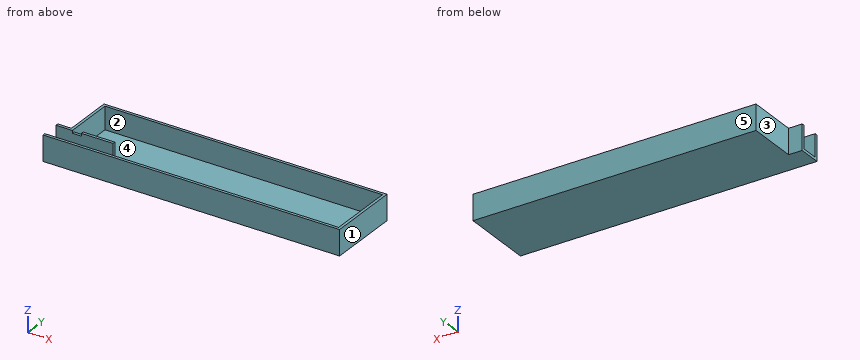
from build123d import *

# Parameters (mm, degrees)
F1_DEPTH = 1.2
F2_W     = 18
F2_H     = 1.2
F3_DEPTH = 10
F4_W     = 4
F4_H     = 1.2
F5_DEPTH = 1.2


with BuildPart() as f1:
    # F0 (on Top) → F1 (new body)
    with BuildSketch(Plane.XY):
        Polygon((-125, 0), (0, 0), (0, 32), (-125, 32), (-125, 10), (-131, 10), (-131, 0), align=None)
    extrude(amount=F1_DEPTH)

    # F2 (on face) → F3 (join)
    with BuildSketch(Plane.XY.offset(1.2)):
        Polygon((-131, 0), (0, 0), (0, 32), (-125, 32), (-125, 10), (-131, 10), (-131, 8.8), (-123.8, 8.8), (-123.8, 10), (-123.8, 30.8), (-1.2, 30.8), (-1.2, 1.2), (-131, 1.2), align=None)
        with Locations((-114.8, 9.4)):
            Rectangle(F2_W, F2_H)
    extrude(amount=F3_DEPTH)

    # F4 (on face) → F5 (cut, through all)
    with BuildSketch(Plane(origin=(0, 10, 0), x_dir=(-1, 0, 0), z_dir=(0, 1, 0))):
        with Locations((121.8, 10.6)):
            Rectangle(F4_W, F4_H)
    extrude(amount=-F5_DEPTH, mode=Mode.SUBTRACT)


solid = f1.part
For this review, take the finished solid that the model builds, in its own axes (mm). Face numbers are marked on the shaded views. A direction names the side the tool comes from. Give positions to 0.01 mm unless a question says otherwise; leave off trailing zeros. Loops run counter-clockwise (first coordinate to the right, second up) from the corner with the lowest first, then second, coordinate; pieces in that order, holes last.
Item 1: Take a section at B-B, the plane y = 15.5. State the section outline as (x, z) points.
Item 2: Take a section at C-C, the plane z = 7.5. State the section outline as (x, y) points, and give its area (3 significant figures).
Item 3: Take a section at A-A, the plane x = -81. State the section outline as (y, z) points.
Item 4: Insertion check: pin 1 (3 mm diameter, centred on y = 13, z = 2.5, fed in from -X); pin 2 (15 mm diameter, centred on x = -63.5, y = 14, fed in from +Z); pin 3 (1 mm diameter, centred on x = -121.5, y = 9.5, fed in from +Z). Each pin has a flat end and moves straight along its axis. Give the tip position at first contact, or say it passes through.
Item 5: Tool access review of the marked faces 1 and 2: name each direction out of +Z, -Z, +X, -X, +Y, -Y from which nothing blocks a thin tool from reaching the whole face with its end or side.
Item 6: For line 1 along Y through (x, z) = (-112.5, 5.5); line 2 along Y through (x, z) = (-41.5, 1.5); line 3 along X through (y, z) = (29, 10), list the stretches that pass through material, from the lowest coordinate up.
Item 7: Draft analysis for pull direction Y (two halves, no side actions). For the marked faces 3, 4 and 5, state which applies: +Y half, -Y half, draft (parallel to the pull), parting line (faces both ways), or undercut.
Item 8: Take a section at D-D, the plane x = -114.5. State the section outline as (y, z) points.
Calculated:
1. outline: (-125, 0) - (0, 0) - (0, 11.2) - (-1.2, 11.2) - (-1.2, 1.2) - (-123.8, 1.2) - (-123.8, 11.2) - (-125, 11.2) - close
2. outline: (-131, 0) - (0, 0) - (0, 32) - (-125, 32) - (-125, 10) - (-131, 10) - (-131, 8.8) - (-105.8, 8.8) - (-105.8, 10) - (-123.8, 10) - (-123.8, 30.8) - (-1.2, 30.8) - (-1.2, 1.2) - (-131, 1.2) - close
2. area: 398 mm2
3. outline: (0, 0) - (32, 0) - (32, 11.2) - (30.8, 11.2) - (30.8, 1.2) - (1.2, 1.2) - (1.2, 11.2) - (0, 11.2) - close
4. pin 1: stops at x = -125
4. pin 2: stops at z = 1.2
4. pin 3: stops at z = 10
5. face 1: +Z, -Z, +X, +Y, -Y
5. face 2: +Z
6. line 1: y = 0 to 1.2, 8.8 to 10, 30.8 to 32
6. line 2: y = 0 to 1.2, 30.8 to 32
6. line 3: x = -125 to -123.8, -1.2 to 0
7. face 3: draft
7. face 4: undercut
7. face 5: +Y half
8. outline: (0, 0) - (32, 0) - (32, 11.2) - (30.8, 11.2) - (30.8, 1.2) - (10, 1.2) - (10, 11.2) - (8.8, 11.2) - (8.8, 1.2) - (1.2, 1.2) - (1.2, 11.2) - (0, 11.2) - close
